Part model, mm, in its own coordinate system. A direction names the side the tool comes from. Round coordinates to 2 decimals unless told otherwise and drop trailing zeros. Order: outer loops, then holes, each group sorted by start corner. A loop starts at its lowest first (then second) coordinate and runs counter-clockwise, first axis right, second up. Notation, with made-up numbers: (11, 61.25) - (62, 61.25) arc R29 cw to (62, 93.25) - close; hole circle Ø10 at (-2.75, 58.5). An arc over 180 degrees is marked (long way). Return JSON: item names as keys, results as strings. Group by question number.
Item 1: Tool access for faces 1 (the face through (-11.808, 0.361, 147.436)), 2 (the face through (-15, -8, 5)), 3 (the face through (-30, 0, 74)): list every direction of +Z, -Z, +X, -X, +Y, -Y with a clear straight run to the whole face (end or side of a thin tool).
Item 2: Saw through at C-C on x = -3.5. List the corners of the cut face in (y, z).
Item 3: Saw through at B-B on x = -20. List the corners of the cut face in (y, z).
Item 4: Saw through at A-A on y = 0. List the corners of the cut face in (x, z).
Item 5: Drop flat-ended pins along their axis: pin 1 (1.9 mm diameter, centred on x = -4, z = 4.5, fed in from +Y); pin 2 (7.5 mm diameter, centred on x = 5, z = 5, fed in from +Y); pin 3 (5 mm diameter, centred on x = 0, y = 0, fed in from +Z). Give the stop position or say it passes through.
Item 6: Saw through at D-D on x = -26.5. List the corners of the cut face in (y, z), and give its area (3 significant figures).
Item 7: Probe probe 1 along X at (y, z) = (5.75, 5); probe 2 along Y at (x, z) = (0, 146.95); probe 3 along Z at (x, y) = (6, -2.75). List the from-to ranges inside material, lowest first.
Item 8: Two-plate mould, pull along Z, no slides. Class faces 4 (the face through (-20, 0, 144.8)), 5 (the face through (-10, -10, 74)), 6 (the face through (-25, -8, 5)): released by +Z, released by -Z, zero draft, split by the parting line, or undercut.
```python
from build123d import *

# Parameters (mm, degrees)
SKETCH_1_W               = 20
SKETCH_1_H               = 20
EXTRUDE_1_DEPTH          = 150
SKETCH_2_R               = 8.2
CUT_EXTRUDE_1_DEPTH      = 5.2
SKETCH_3_R               = 3.2
CUT_EXTRUDE_2_DEPTH      = 18
MIRROR_2_COPY_1_SKETCH_R = 3.2
MIRROR_2_COPY_1_DEPTH    = 18


with BuildPart() as part:
    # ｽｹｯﾁ1 → ﾎﾞｽ - 押し出し1 (new body)
    with BuildSketch(Plane.XY):
        Rectangle(SKETCH_1_W, SKETCH_1_H)
    extrude_1 = extrude(amount=EXTRUDE_1_DEPTH)

    # ｽｹｯﾁ2 → ｶｯﾄ - 押し出し1 (cut)
    with BuildSketch(Plane.XY.offset(150)):
        Circle(SKETCH_2_R)
    cut_extrude_1 = extrude(amount=-CUT_EXTRUDE_1_DEPTH, mode=Mode.SUBTRACT)

    # ｽｹｯﾁ3 → ｶｯﾄ - 押し出し2 (cut)
    with BuildSketch(Plane(origin=(0, 10, 0), x_dir=(1, 0, 0), z_dir=(0, 1, 0))):
        with Locations(Location((5, -5, 0), (0, 0, 270))):
            Circle(SKETCH_3_R)
    cut_extrude_2 = extrude(amount=-CUT_EXTRUDE_2_DEPTH, mode=Mode.SUBTRACT)

    # ﾐﾗｰ1: ｶｯﾄ - 押し出し2 across plane
    add(cut_extrude_2.mirror(Plane(origin=(0, 0, 0), x_dir=(0, 0, 1), z_dir=(1, 0, 0))), mode=Mode.SUBTRACT)

    # ﾐﾗｰ2: ﾎﾞｽ - 押し出し1, ｶｯﾄ - 押し出し1, ｶｯﾄ - 押し出し2 across plane
    add(extrude_1.mirror(Plane(origin=(-10, 10, 150), x_dir=(0, 0, 1), z_dir=(1, 0, 0))))
    add(cut_extrude_1.mirror(Plane(origin=(-10, 10, 150), x_dir=(0, 0, 1), z_dir=(1, 0, 0))), mode=Mode.SUBTRACT)
    add(cut_extrude_2.mirror(Plane(origin=(-10, 10, 150), x_dir=(0, 0, 1), z_dir=(1, 0, 0))), mode=Mode.SUBTRACT)

    # ﾐﾗｰ2 copy 1 sketch → ﾐﾗｰ2 copy 1 (cut)
    with BuildSketch(Plane(origin=(-20, 10, 0), x_dir=(1, 0, 0), z_dir=(0, 1, 0))):
        with Locations(Location((5, -5, 0), (0, 0, 270))):
            Circle(MIRROR_2_COPY_1_SKETCH_R)
    extrude(amount=-MIRROR_2_COPY_1_DEPTH, mode=Mode.SUBTRACT)


solid = part.part
```
Filled in:
{
 "1": {"face 1": "+Z", "face 2": "+Y", "face 3": "+Z, -Z, -X, +Y, -Y"},
 "2": {"outline": "(-10, 0) - (10, 0) - (10, 2.17) - (-8, 2.17) - (-8, 7.83) - (10, 7.83) - (10, 150) - (7.42, 150) - (7.42, 144.8) - (-7.42, 144.8) - (-7.42, 150) - (-10, 150) - close"},
 "3": {"outline": "(-10, 0) - (10, 0) - (10, 150) - (8.2, 150) - (8.2, 144.8) - (-8.2, 144.8) - (-8.2, 150) - (-10, 150) - close"},
 "4": {"outline": "(-30, 0) - (10, 0) - (10, 150) - (8.2, 150) - (8.2, 144.8) - (-8.2, 144.8) - (-8.2, 150) - (-11.8, 150) - (-11.8, 144.8) - (-28.2, 144.8) - (-28.2, 150) - (-30, 150) - close; hole circle Ø6.4 at (-25, 5); hole circle Ø6.4 at (-15, 5); hole circle Ø6.4 at (-5, 5); hole circle Ø6.4 at (5, 5)"},
 "5": {"pin 1": "stops at y = -8", "pin 2": "stops at y = 10", "pin 3": "stops at z = 144.8"},
 "6": {"outline": "(-10, 0) - (10, 0) - (10, 2.17) - (-8, 2.17) - (-8, 7.83) - (10, 7.83) - (10, 150) - (5, 150) - (5, 144.8) - (-5, 144.8) - (-5, 150) - (-10, 150) - close", "area": "2,850 mm^2"},
 "7": {"probe 1": "x = -30 to -28.2, -21.8 to -18.2, -11.8 to -8.2, -1.8 to 1.8, 8.2 to 10", "probe 2": "y = -10 to -8.2, 8.2 to 10", "probe 3": "z = 0 to 1.96, 8.04 to 144.8"},
 "8": {"face 4": "released by +Z", "face 5": "zero draft", "face 6": "undercut"}
}
